from build123d import *

# Parameters (mm, degrees)
SKETCH1_W           = 83.82
SKETCH1_H           = 27.225
BOSS_EXTRUDE1_DEPTH = 87.122
SHELL1_T            = -2.54
SKETCH12_W          = 83.82
SKETCH12_H          = 27.225
BOSS_EXTRUDE6_DEPTH = 46.99
SHELL2_START        = 2.54
SHELL2_OUTLINE_W    = 44.45
SHELL2_OUTLINE_H    = 24.685
SHELL2_DEPTH        = 78.74
SKETCH5_R           = 3.175
SKETCH5_R_2         = 1.5
BOSS_EXTRUDE7_DEPTH = 1.905
CUT_EXTRUDE10_REACH = 162.477
SKETCH14_W          = 16.764
SKETCH14_H          = 12.192
SKETCH15_W          = 30.48
SKETCH15_H          = 46.99
BOSS_EXTRUDE8_DEPTH = 10.16
SKETCH16_W          = 7.62
SKETCH16_H          = 41.91
CUT_EXTRUDE11_DEPTH = 161.477479943
CHAMFER1_SIZE       = 5.08
SKETCH17_R          = 1.5
CUT_EXTRUDE12_DEPTH = 10
FILLET1_R           = 3


# Read off the part's stored shape, not the designer's step: Shell2
with BuildPart() as part:
    # Sketch1 → Boss-Extrude1 (new body)
    with BuildSketch(Plane(origin=(0, 0, 0), x_dir=(1, 0, 0), z_dir=(0, 1, 0))):
        with Locations((41.91, 13.6125)):
            Rectangle(SKETCH1_W, SKETCH1_H)
    extrude(amount=BOSS_EXTRUDE1_DEPTH)

    # Shell1
    shell1_openings = [part.faces().sort_by_distance(p)[0] for p in [
        (41.91, 43.561, -27.225),
    ]]
    offset(amount=SHELL1_T, openings=shell1_openings, kind=Kind.INTERSECTION)

    # Sketch12 → Boss-Extrude6 (add)
    with BuildSketch(Plane(origin=(0, 87.122, 0), x_dir=(1, 0, 0), z_dir=(0, 1, 0))):
        with Locations((41.91, 13.6125)):
            Rectangle(SKETCH12_W, SKETCH12_H)
    extrude(amount=BOSS_EXTRUDE6_DEPTH)

    # Shell2 outline → Shell2 (cut)
    with BuildSketch(Plane.YZ.offset(SHELL2_START)):
        with Locations((109.347, -14.8825)):
            Rectangle(SHELL2_OUTLINE_W, SHELL2_OUTLINE_H)
    extrude(amount=SHELL2_DEPTH, mode=Mode.SUBTRACT)

    # Sketch5 → Boss-Extrude7 (add)
    # profile 1 of 4: a face of its own
    with BuildSketch(Plane(origin=(0, 88.392, -2.54), x_dir=(1, 0, 0), z_dir=(0, 0, -1))):
        with Locations((15.24, -29.845)):
            Circle(SKETCH5_R)
        with Locations((15.24, -29.845)):
            Circle(SKETCH5_R_2, mode=Mode.SUBTRACT)
    # profile 2 of 4: a face of its own
    with BuildSketch(Plane(origin=(0, 88.392, -2.54), x_dir=(1, 0, 0), z_dir=(0, 0, -1))):
        with Locations((15.24, -9.525)):
            Circle(SKETCH5_R)
        with Locations((15.24, -9.525)):
            Circle(SKETCH5_R_2, mode=Mode.SUBTRACT)
    # profile 3 of 4: a face of its own
    with BuildSketch(Plane(origin=(0, 88.392, -2.54), x_dir=(1, 0, 0), z_dir=(0, 0, -1))):
        with Locations((49.53, -9.525)):
            Circle(SKETCH5_R)
        with Locations((49.53, -9.525)):
            Circle(SKETCH5_R_2, mode=Mode.SUBTRACT)
    # profile 4 of 4: a face of its own
    with BuildSketch(Plane(origin=(0, 88.392, -2.54), x_dir=(1, 0, 0), z_dir=(0, 0, -1))):
        with Locations((49.53, -29.845)):
            Circle(SKETCH5_R)
        with Locations((49.53, -29.845)):
            Circle(SKETCH5_R_2, mode=Mode.SUBTRACT)
    extrude(amount=BOSS_EXTRUDE7_DEPTH)

    # Sketch14 → Cut-Extrude10 (cut, up to next)
    with BuildSketch(Plane(origin=(0, 134.112, 0), x_dir=(1, 0, 0), z_dir=(0, 1, 0)), mode=Mode.PRIVATE) as cut_extrude10_sk1:
        with Locations((41.91, 17.78)):
            Rectangle(SKETCH14_W, SKETCH14_H)
    cut_extrude10_tool1 = extrude(cut_extrude10_sk1.sketch, amount=-CUT_EXTRUDE10_REACH, mode=Mode.PRIVATE) & part.part
    add(cut_extrude10_tool1.solids().sort_by_distance((41.91, 134.112, -17.78))[0], mode=Mode.SUBTRACT)

    # Sketch15 → Boss-Extrude8 (add)
    with BuildSketch(Plane.XY):
        with Locations((15.24, 110.617)):
            Rectangle(SKETCH15_W, SKETCH15_H)
        with Locations((68.58, 110.617)):
            Rectangle(SKETCH15_W, SKETCH15_H)
    extrude(amount=BOSS_EXTRUDE8_DEPTH)

    # Sketch16 → Cut-Extrude11 (cut, through all)
    with BuildSketch(Plane.ZY):
        with Locations((3.81, 110.617)):
            Rectangle(SKETCH16_W, SKETCH16_H)
    extrude(amount=-CUT_EXTRUDE11_DEPTH, mode=Mode.SUBTRACT)

    # Chamfer1
    chamfer1_edges = [part.edges().sort_by_distance(p)[0] for p in [
        (2.54, 2.54, -14.8825),
        (81.28, 2.54, -14.8825),
        (2.54, 84.582, -14.8825),
        (81.28, 84.582, -14.8825),
    ]]
    chamfer(chamfer1_edges, length=CHAMFER1_SIZE)

    # Sketch17 → Cut-Extrude12 (cut)
    with BuildSketch(Plane(origin=(0, 0, -27.225), x_dir=(-1, 0, 0), z_dir=(0, 0, -1))):
        with Locations((-3, 84.122)):
            Circle(SKETCH17_R)
        with Locations((-80.82, 84.122)):
            Circle(SKETCH17_R)
        with Locations((-80.82, 3)):
            Circle(SKETCH17_R)
        with Locations((-3, 3)):
            Circle(SKETCH17_R)
    extrude(amount=-CUT_EXTRUDE12_DEPTH, mode=Mode.SUBTRACT)

    # Fillet1
    # the kernel refuses this fillet: 3 mm, written as the material it takes off along each edge
    with BuildSketch(Plane(origin=(91.32, 134.112, 10.16), x_dir=(0, 0, -1), z_dir=(-1, 0, 0)), Plane(origin=(45.84, 87.122, 10.16), x_dir=(0, 0, -1), z_dir=(1, 0, 0)), Plane(origin=(37.98, 87.122, 10.16), x_dir=(0, 1, 0), z_dir=(-1, 0, 0))) as fillet1_piece_1:
        with BuildLine():
            CenterArc((FILLET1_R, FILLET1_R), FILLET1_R, 180, 90)
            Line((0, FILLET1_R), (0, 0))
            Line((0, 0), (FILLET1_R, 0))
        make_face()
    extrude(amount=45.48, mode=Mode.SUBTRACT)
    with BuildSketch(Plane(origin=(-7.5, 134.112, 10.16), x_dir=(0, 0, -1), z_dir=(1, 0, 0))) as fillet1_piece_2:
        with BuildLine():
            CenterArc((FILLET1_R, -FILLET1_R), FILLET1_R, 90, 90)
            Line((0, -FILLET1_R), (0, 0))
            Line((0, 0), (FILLET1_R, 0))
        make_face()
    extrude(amount=45.48, mode=Mode.SUBTRACT)
    with BuildSketch(Plane(origin=(83.82, 134.112, -34.725), x_dir=(0, -1, 0), z_dir=(0, 0, 1))) as fillet1_piece_3:
        with BuildLine():
            CenterArc((FILLET1_R, -FILLET1_R), FILLET1_R, 90, 90)
            Line((0, -FILLET1_R), (0, 0))
            Line((0, 0), (FILLET1_R, 0))
        make_face()
    extrude(amount=52.385, mode=Mode.SUBTRACT)
    with BuildSketch(Plane(origin=(83.82, 0, 7.5), x_dir=(0, 1, 0), z_dir=(0, 0, -1))) as fillet1_piece_4:
        with BuildLine():
            CenterArc((FILLET1_R, -FILLET1_R), FILLET1_R, 90, 90)
            Line((0, -FILLET1_R), (0, 0))
            Line((0, 0), (FILLET1_R, 0))
        make_face()
    extrude(amount=42.225, mode=Mode.SUBTRACT)
    with BuildSketch(Plane(origin=(0, 0, -34.725), x_dir=(1, 0, 0), z_dir=(0, 0, 1))) as fillet1_piece_5:
        with BuildLine():
            CenterArc((FILLET1_R, FILLET1_R), FILLET1_R, 180, 90)
            Line((0, FILLET1_R), (0, 0))
            Line((0, 0), (FILLET1_R, 0))
        make_face()
    extrude(amount=42.225, mode=Mode.SUBTRACT)
    with BuildSketch(Plane(origin=(0, 134.112, 17.66), x_dir=(1, 0, 0), z_dir=(0, 0, -1))) as fillet1_piece_6:
        with BuildLine():
            CenterArc((FILLET1_R, FILLET1_R), FILLET1_R, 180, 90)
            Line((0, FILLET1_R), (0, 0))
            Line((0, 0), (FILLET1_R, 0))
        make_face()
    extrude(amount=52.385, mode=Mode.SUBTRACT)


solid = part.part
Geometry check sheet. Reference: the model listing, model coordinates, mm. A direction names the side the tool comes from. Round coordinates to 2 decimals unless told otherwise and drop trailing zeros. Write each loop counter-clockwise with the first axis right and the second up, starting at its lowest first coordinate (ties: lowest second). Pieces come first, ordered by that corner, then holes.
Item 1: Section check B-B (x = 64.5). Record the boundary of the cut face in (y, z) (3 decimals).
Determined:
outline: (0, -27.225) - (2.54, -27.225) - (2.54, -2.54) - (84.582, -2.54) - (84.582, -27.225) - (87.122, -27.225) - (87.122, -2.54) - (131.572, -2.54) - (131.572, -27.225) - (134.112, -27.225) - (134.112, 7.16) arc R3 ccw to (131.112, 10.16) - (90.122, 10.16) arc R3 ccw to (87.122, 7.16) - (87.122, 0) - (0, 0) - close; hole (89.662, 0) - (131.572, 0) - (131.572, 7.62) - (89.662, 7.62) - close
Item 2: Go/stop test with flat-tipped pins: pin 1 Ø3 at (x, z) = (41.5, -23.5) entering from -Y; pin 2 Ø2.5 at (x, y) = (14.5, 117.5) entering from -Z (3 decimals); pin 3 Ø9 at (x, y) = (9, 109) entering from -Z; pin 4 Ø2.5 at (x, y) = (80.82, 3) entering from -Z (3 decimals). Record where each tip stops, or that it passes through.
Determined:
pin 1: stops at y = 0
pin 2: stops at z = -4.445
pin 3: stops at z = -2.54
pin 4: stops at z = -17.225
Item 3: Section check D-D (z = -19). Record the boundary of the cut face in (x, y).
Determined:
outline: (0, 3) arc R3 ccw to (3, 0) - (80.82, 0) arc R3 ccw to (83.82, 3) - (83.82, 131.11) arc R3 ccw to (80.82, 134.11) - (50.29, 134.11) - (50.29, 131.57) - (81.28, 131.57) - (81.28, 87.12) - (2.54, 87.12) - (2.54, 131.57) - (33.53, 131.57) - (33.53, 134.11) - (3, 134.11) arc R3 ccw to (0, 131.11) - close; hole circle Ø3 at (3, 3); hole circle Ø3 at (3, 84.12); hole (2.54, 7.62) - (7.62, 2.54) - (76.2, 2.54) - (81.28, 7.62) - (81.28, 79.5) - (76.2, 84.58) - (7.62, 84.58) - (2.54, 79.5) - close; hole circle Ø3 at (80.82, 3); hole circle Ø3 at (80.82, 84.12)
Item 4: Material ranges on line 1 along Y through (x, z) = (51.5, -21); line 2 along X through (y, z) = (14.5, -22); line 3 along Y through (x, z) = (76.5, -18), recorded low to high.
Determined:
line 1: y = 0 to 2.54, 84.58 to 87.12, 131.57 to 134.11
line 2: x = 0 to 2.54, 81.28 to 83.82
line 3: y = 0 to 2.84, 84.28 to 87.12, 131.57 to 134.11
Item 5: Section check C-C (y = 105). Record the boundary of the cut face in (x, z) (3 decimals).
Determined:
outline: (0, -27.225) - (2.54, -27.225) - (2.54, -2.54) - (81.28, -2.54) - (81.28, -27.225) - (83.82, -27.225) - (83.82, 0) - (0, 0) - close; (0, 7.62) - (30.48, 7.62) - (30.48, 10.16) - (0, 10.16) - close; (53.34, 7.62) - (83.82, 7.62) - (83.82, 10.16) - (53.34, 10.16) - close
Item 6: Mould release check, pull along Z, two halves, no side actions. Record for faces 1 (the face through (33.528, 133, -18)), 2 (the face through (68.793, 133.21, 9.305)), 3 (the face through (53.34, 109, 8)): +Z half, -Z half, draft (parallel to the pull), parting line (faces both ways), or undercut.
Determined:
face 1: undercut
face 2: +Z half
face 3: draft
Item 7: Access from +Z, -Z, +X, -X, +Y, -Y to the whole of each face (thin tool, end or side, straight path). Record for faces 4 (the face through (50.292, 133, -18)), 5 (the face through (51.24, 115.56, -3.48)), 6 (the face through (68, 131.572, 4)).
Determined:
face 4: +Y
face 5: -Z
face 6: +X, -X
Item 8: Section check A-A (z = 2). Record the boundary of the cut face in (x, y), plus the area to 3 significant figures.
Determined:
outline: (0, 87.12) - (30.48, 87.12) - (30.48, 89.66) - (0, 89.66) - close; (0.04, 131.57) - (30.48, 131.57) - (30.48, 134.11) - (3, 134.11) arc R3 ccw to start; (53.34, 87.12) - (83.82, 87.12) - (83.82, 89.66) - (53.34, 89.66) - close; (53.34, 131.57) - (83.78, 131.57) arc R3 ccw to (80.82, 134.11) - (53.34, 134.11) - close
area: 306 mm2
